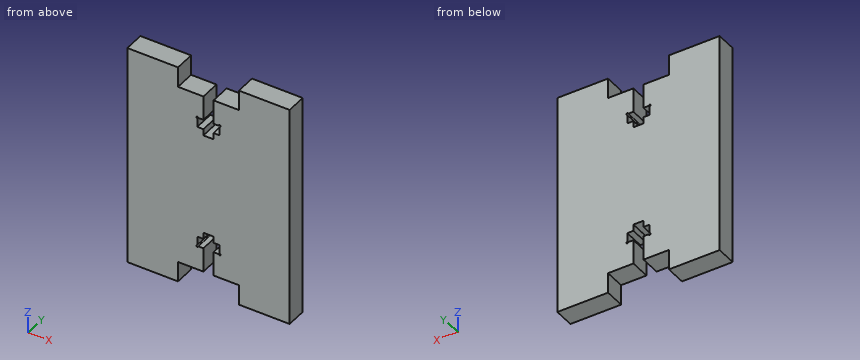
```python
from build123d import *

# Parameters (mm, degrees)
SCHIZZO1_W                   = 40
SCHIZZO1_H                   = 55
ESTRUSIONE_ESTRUSIONE2_DEPTH = 5
SCHIZZO2_W                   = 15
SCHIZZO2_H                   = 5
TAGLIO_ESTRUSIONE1_DEPTH     = 6
TAGLIO_ESTRUSIONE3_DEPTH     = 6
SCHIZZO4_R                   = 0.25
TAGLIO_ESTRUSIONE4_DEPTH     = 10


with BuildPart() as part:
    # Schizzo1 → Estrusione-Estrusione2 (new body)
    with BuildSketch(Plane(origin=(0, 0, 0), x_dir=(1, 0, 0), z_dir=(0, 1, 0))):
        with Locations((-34.56494914, -0.781075862)):
            Rectangle(SCHIZZO1_W, SCHIZZO1_H)
    extrude(amount=-ESTRUSIONE_ESTRUSIONE2_DEPTH)

    # Schizzo2 → Taglio-Estrusione1 (cut, through all)
    with BuildSketch(Plane(origin=(0, 0, 0), x_dir=(1, 0, 0), z_dir=(0, 1, 0))):
        with Locations((-34.56494914, -25.781075862)):
            Rectangle(SCHIZZO2_W, SCHIZZO2_H)
        with Locations((-34.56494914, 24.218924138)):
            Rectangle(SCHIZZO2_W, SCHIZZO2_H)
    extrude(amount=-TAGLIO_ESTRUSIONE1_DEPTH, mode=Mode.SUBTRACT)

    # Schizzo3 → Taglio-Estrusione3 (cut, through all)
    with BuildSketch(Plane(origin=(0, 0, 0), x_dir=(1, 0, 0), z_dir=(0, 1, 0))):
        Polygon((-35.81494914, -23.281075862), (-33.31494914, -23.281075862), (-33.31494914, -17.281075862), (-31.81494914, -17.281075862), (-31.81494914, -14.881075862), (-33.31494914, -14.881075862), (-33.31494914, -13.281075862), (-35.81494914, -13.281075862), (-35.81494914, -14.881075862), (-37.31494914, -14.881075862), (-37.31494914, -17.281075862), (-35.81494914, -17.281075862), align=None)
        Polygon((-35.81494914, 11.718924138), (-33.31494914, 11.718924138), (-33.31494914, 13.318924138), (-31.81494914, 13.318924138), (-31.81494914, 15.718924138), (-33.31494914, 15.718924138), (-33.31494914, 21.718924138), (-35.81494914, 21.718924138), (-35.81494914, 15.718924138), (-37.31494914, 15.718924138), (-37.31494914, 13.318924138), (-35.81494914, 13.318924138), align=None)
    extrude(amount=-TAGLIO_ESTRUSIONE3_DEPTH, mode=Mode.SUBTRACT)

    # Schizzo4 → Taglio-Estrusione4 (cut)
    with BuildSketch(Plane(origin=(0, 0, 0), x_dir=(1, 0, 0), z_dir=(0, 1, 0))):
        with Locations((-37.31494914, -17.281075862)):
            Circle(SCHIZZO4_R)
        with Locations((-31.81494914, -17.281075862)):
            Circle(SCHIZZO4_R)
        with Locations((-37.31494914, 15.718924138)):
            Circle(SCHIZZO4_R)
        with Locations((-31.81494914, 15.718924138)):
            Circle(SCHIZZO4_R)
    extrude(amount=-TAGLIO_ESTRUSIONE4_DEPTH, mode=Mode.SUBTRACT)


solid = part.part
```
Verification items for the finished model (mm, model axes). Coordinates: 2 decimals unless noted, no trailing zeros. Write each loop counter-clockwise with the first axis right and the second up, starting at its lowest first coordinate (ties: lowest second). Pieces come first, ordered by that corner, then holes. Notation, with made-up numbers: M 28,-20 L 77,-20 A23 ccw 77,9 Z; hole C 1.5,-21 d7. An arc over 180 degrees is marked long. One line per item, written item: value.
Item 1: Scan lines: line 1 along X through (y, z) = (-3.6, 18.5); line 2 along X through (y, z) = (-1.4, 25); line 3 along Z through (x, y) = (-32, -3.45). Record each from-to range of solid material in increasing order.
Check sheet entries:
line 1: x = -54.56 to -35.81, -33.31 to -14.56
line 2: x = -54.56 to -42.06, -27.06 to -14.56
line 3: z = -21.72 to -15.89, -13.32 to 14.88, 17.45 to 23.28
Item 2: Section check B-B, the plane x = -39. Record the boundary of the cut face in (y, z), plus the area to 3 significant figures.
Check sheet entries:
outline: M -5,-21.72 L 0,-21.72 L 0,23.28 L -5,23.28 Z
area: 225 mm^2
Item 3: Section check A-A, the plane x = -34. Record the boundary of the cut face in (y, z).
Check sheet entries:
outline: M -5,-11.72 L 0,-11.72 L 0,13.28 L -5,13.28 Z
Item 4: Gauge pin test, flat ends, axial feed: pin 1 Ø0.8 at (x, y) = (-34.5, -1.5) entering from -Z; pin 2 Ø0.8 at (x, y) = (-32.5, -2) entering from +Z; pin 3 Ø1 at (x, y) = (-33, -2.5) entering from -Z. Record the tip position at first contact, or that the pin passes through.
Check sheet entries:
pin 1: stops at z = -11.72
pin 2: stops at z = 23.28
pin 3: stops at z = -21.72
